Could you check a few things on this model? Use its own coordinates, in mm. Face numbers are marked on the shaded views. A direction names the side the tool comes from. Coordinates: 2 decimals unless noted, no trailing zeros. Order: outer loops, then holes, each group sorted by start corner. A loop starts at its lowest first (then second) coordinate and runs counter-clockwise, first axis right, second up. Notation, with made-up numbers: (81.25, 41) -> (97.25, 41) arc R16 ccw to (97.25, 70) -> close; hole circle Ø11 at (62, 7). An arc over 180 degrees is marked (long way). Use a Markdown table: item, result. Add a question column.
1) If I drill on L1, parallel to X at y = -9.5, z = 9.5; L2, parallel to X at y = -5.25, z = 16.5; L3, parallel to Z at x = -4.5, y = -3.5, over which ranges is the centre line in solid material (lowest first)? Write a range as [from, to].
2) Which directions (+Z, -Z, +X, -X, +Y, -Y) give clear straight access to the entire face, cutting with the end or side of a thin tool? Please do the marked faces 4 and 5.
3) If we section it at D-D (z = 17): Write out the boundary of the cut face in (x, y), plus the area to 3 significant figures.
4) If we section it at B-B (z = 10.25): Write out the boundary of the cut face in (x, y), plus the area to 3 significant figures.
5) If we section it at C-C (y = -6): Write out the boundary of the cut face in (x, z), plus the area to 3 significant figures.
6) Will these pins go through, and if not, where does the flat tip stop? pin 1 Ø4.5 at (y, z) = (-5.5, 11.5) entering from +X; pin 2 Ø2.5 at (y, z) = (-6.5, 7) entering from -X; pin 3 Ø2 at (x, y) = (-1.5, -1) entering from +Z; pin 4 Ø6 at (x, y) = (-3.5, -4.5) entering from -Z.
7) If we section it at A-A (z = 13): Write out the boundary of the cut face in (x, y), plus the area to 3 significant figures.
8) Thinking about a two-plate mould opening in Z: for the marked faces 1, 2 and 3, which applies, +Z half, -Z half, draft (parallel to the pull), parting line (faces both ways), or undercut?
```python
from build123d import *

# Parameters (mm, degrees)
PAD_DEPTH       = 10
POCKET_DEPTH    = 10.001
SKETCH002_R     = 2.749127
POCKET001_DEPTH = 12.55872
FILLET_R        = 3


with BuildPart() as part:
    # Sketch → Pad (new body)
    with BuildSketch(Plane.XZ):
        with BuildLine():
            ThreePointArc((4.409319, 13.530378), (0, 28.531103), (-4.409319, 13.530378))
            Line((-4.409319, 13.530378), (-4.409319, 4.742104))
            Line((-4.409319, 4.742104), (4.409319, 4.742104))
            Line((4.409319, 4.742104), (4.409319, 13.530378))
        make_face()
    extrude(amount=PAD_DEPTH)

    # Sketch001 → Pocket (cut, through all)
    with BuildSketch(Plane.XZ):
        with BuildLine():
            ThreePointArc((4.186002, 13.626635), (0, 28.346632), (-4.186002, 13.626635))
            Line((-4.186002, 13.626635), (-4.186002, 4.191096))
            Line((-4.186002, 4.191096), (4.186002, 4.191096))
            Line((4.186002, 4.191096), (4.186002, 13.626635))
        make_face()
    extrude(amount=POCKET_DEPTH, mode=Mode.SUBTRACT)

    # Sketch002 (on Face2 of Pocket) → Pocket001 (cut, through all)
    with BuildSketch(Plane(origin=(4.409319, 0, 0), x_dir=(0, 0, 1), z_dir=(1, 0, 0))):
        with Locations((9.13458, 4.909179)):
            Circle(SKETCH002_R)
    extrude(amount=-POCKET001_DEPTH, mode=Mode.SUBTRACT)

    # Fillet
    fillet_edges = [part.edges().sort_by_distance(p)[0] for p in [
        (4.297661, -10, 4.742104),
        (-4.297661, -10, 4.742104),
        (-4.297661, 0, 4.742104),
        (4.297661, 0, 4.742104),
    ]]
    fillet(fillet_edges, radius=FILLET_R)


solid = part.part
```
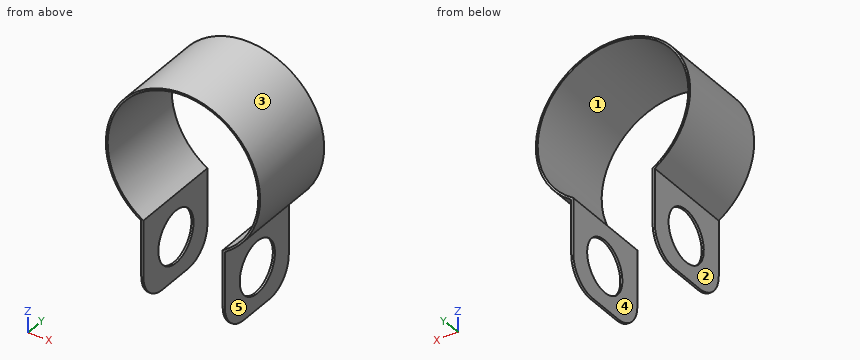
Answer sheet:
| question | item | result |
|---|---|---|
| 1 | L1 | [-4.41, -4.19], [4.19, 4.41] |
| 1 | L2 | [-7.16, -6.94], [6.94, 7.16] |
| 1 | L3 | [13.59, 13.83], [26.95, 27.18] |
| 2 | face 4 | -Z, +Y, -Y |
| 2 | face 5 | -Z, +X, +Y, -Y |
| 3 | outline | (-7.41, -10) -> (-7.2, -10) -> (-7.2, 0) -> (-7.41, 0) -> close; (7.2, -10) -> (7.41, -10) -> (7.41, 0) -> (7.2, 0) -> close |
| 3 | area | 4.34 mm2 |
| 4 | outline | (-4.41, -10) -> (-4.19, -10) -> (-4.19, -7.42) -> (-4.41, -7.42) -> close; (-4.41, -2.4) -> (-4.19, -2.4) -> (-4.19, 0) -> (-4.41, 0) -> close; (4.19, -10) -> (4.41, -10) -> (4.41, -7.42) -> (4.19, -7.42) -> close; (4.19, -2.4) -> (4.41, -2.4) -> (4.41, 0) -> (4.19, 0) -> close |
| 4 | area | 2.22 mm2 |
| 5 | outline | (-4.41, 4.74) -> (-4.19, 4.74) -> (-4.19, 6.61) -> (-4.41, 6.61) -> close; (-4.41, 11.66) -> (-4.19, 11.66) -> (-4.19, 13.63) arc R7.96 cw (long way) to (4.19, 13.63) -> (4.19, 11.66) -> (4.41, 11.66) -> (4.41, 13.53) arc R8.15 ccw (long way) to (-4.41, 13.53) -> close; (4.19, 4.74) -> (4.41, 4.74) -> (4.41, 6.61) -> (4.19, 6.61) -> close |
| 5 | area | 9.64 mm2 |
| 6 | pin 1 | x = 4.73 |
| 6 | pin 2 | x = -4.41 |
| 6 | pin 3 | z = 28.52 |
| 6 | pin 4 | z = 4.74 |
| 7 | outline | (-4.41, -10) -> (-4.19, -10) -> (-4.19, 0) -> (-4.41, 0) -> close; (4.19, -10) -> (4.41, -10) -> (4.41, 0) -> (4.19, 0) -> close |
| 7 | area | 4.47 mm2 |
| 8 | face 1 | undercut |
| 8 | face 2 | draft |
| 8 | face 3 | parting line |
